Check sheet for the modelled part. Datum: model origin and axes. Units: mm. Give positions to 0.01 mm unless a question says otherwise; leave off trailing zeros. Write each loop counter-clockwise with the first axis right and the second up, starting at its lowest first coordinate (ties: lowest second). Pieces come first, ordered by that corner, then holes. Notation, with made-up numbers: M 64,27.5 L 74,27.5 A11 ccw 74,31.5 Z; hole C -37,-24.5 d8. An arc over 180 degrees is marked long. Write item = value, one per line. Start each with the question number.
1) Sectioned sample at B-B, the plane x = -272.5. Record the cut outline in (y, z).
2) Sectioned sample at C-C, the plane z = 493.5. Record the cut outline in (x, y), then the cut area to 3 significant figures.
3) Gauge pin test, flat ends, axial feed: pin 1 (25 mm diameter, centred on x = 36.5, z = 521.5, fed in from +Y); pin 2 (25 mm diameter, centred on y = -0.5, z = 1515.5, fed in from +X); pin 3 (15 mm diameter, centred on y = 1.5, z = 1329, fed in from -X); pin 4 (12 mm diameter, centred on y = -294, z = 446.5, fed in from -X). Record the tip position at first contact, or that the pin passes through.
4) Sectioned sample at A-A, the plane y = -48. Record the cut outline in (x, z), then the cut area to 3 significant figures.
5) Sectioned sample at D-D, the plane z = 1471. Record the cut outline in (x, y), then the cut area to 3 significant figures.
6) Scan lines: L1, parallel to X at y = 22, z = 203.5; L2, parallel to Z at x = 211, y = -1.5; L3, parallel to Z at x = -124, y = -15.5. Record each from-to range of solid material in increasing order.
from build123d import *

# Parameters (mm, degrees)
F1_DEPTH  = 25
F3_DEPTH  = 50
F1_FACE_W = 50
F1_FACE_H = 50
F4_DEPTH  = 1000


with BuildPart() as f1:
    # F0 (on Front) → F1 (new body, symmetric)
    with BuildSketch(Plane.XZ):
        Polygon((-475, 0), (0, 0), (50, 0), (525, 0), (525, 50), (50, 929.985795), (50, 1000), (0, 1000), (0, 929.985795), (-475, 50), align=None)
        Polygon((0, 824.722637), (0, 50), (-418.180901, 50), align=None, mode=Mode.SUBTRACT)
        Polygon((468.180901, 50), (50, 50), (50, 824.722637), align=None, mode=Mode.SUBTRACT)
    extrude(amount=F1_DEPTH, both=True)

    # F2 (on Right) → F3 (join)
    with BuildSketch(Plane.YZ):
        Polygon((-500, 50), (-500, 0), (500, 0), (500, 50), (25, 929.985795), (-25, 929.985795), align=None)
        Polygon((-25, 50), (-443.180901, 50), (-25, 824.722637), align=None, mode=Mode.SUBTRACT)
        Polygon((25, 50), (25, 824.722637), (443.180901, 50), align=None, mode=Mode.SUBTRACT)
    extrude(amount=F3_DEPTH)

    # F1_face (on face) → F4 (join)
    with BuildSketch(Plane(origin=(25, 0, 1000), x_dir=(1, 0, 0), z_dir=(0, 0, 1))):
        Rectangle(F1_FACE_W, F1_FACE_H)
    extrude(amount=F4_DEPTH)


solid = f1.part
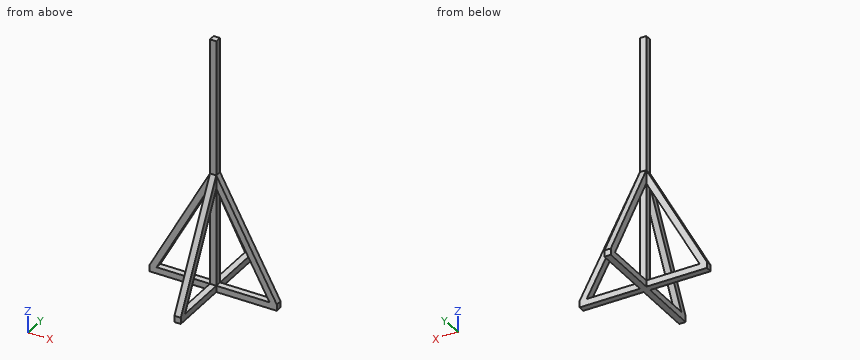
Data:
q1.outline = M -25,0 L 25,0 L 25,50 L -25,50 Z; M -25,319.89 L 25,319.89 L 25,425.15 L -25,425.15 Z
q2.outline = M -235.61,-25 L -178.79,-25 L -178.79,25 L -235.61,25 Z; M 0,-260.61 L 50,-260.61 L 50,-203.79 L 0,-203.79 Z; M 0,-25 L 50,-25 L 50,25 L 0,25 Z; M 0,203.79 L 50,203.79 L 50,260.61 L 0,260.61 Z; M 228.79,-25 L 285.61,-25 L 285.61,25 L 228.79,25 Z
q2.area = 13,900 mm2
q3.pin_1 = 252.24
q3.pin_2 = 50
q3.pin_3 = 0
q3.pin_4 = through
q4.outline = M 0,0 L 50,0 L 50,50 L 0,50 Z; M 0,782.11 L 50,782.11 L 50,887.38 L 0,887.38 Z
q4.area = 7,760 mm2
q5.outline = M 0,-25 L 50,-25 L 50,25 L 0,25 Z
q5.area = 2,500 mm2
q6.L1 = -392.14 to -335.32, 0 to 50, 385.32 to 442.14
q6.L2 = 0 to 50, 526.45 to 631.72
q6.L3 = 0 to 50, 595 to 700.26
